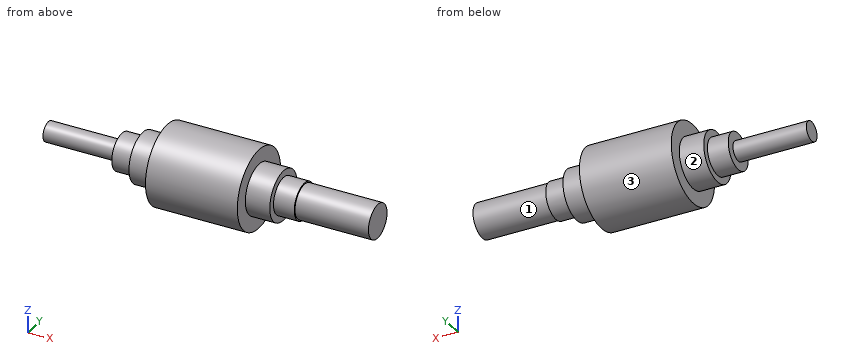
from build123d import *


with BuildPart() as part:
    # Çizim1 → Döndür1 (revolve)
    with BuildSketch(Plane.XY, mode=Mode.PRIVATE) as d_nd_r1_sk:
        Polygon((30, 7.5), (38.5, 7.5), (38.5, 10.25), (48.5, 10.25), (48.5, 16.275), (86, 16.275), (86, 10.25), (96, 10.25), (96, 7.5), (104.5, 7.5), (104.5, 6.975), (134.5, 6.975), (134.5, 0), (0, 0), (0, 4), (30, 4), align=None)
    revolve(d_nd_r1_sk.sketch.rotate(Axis((0, 0, 0), (1, 0, 0)), 90), axis=Axis((0, 0, 0), (1, 0, 0)))


solid = part.part
Work out the finished part from the listing and answer in its coordinate system (mm). Face numbers are marked on the shaded views. A direction names the side the tool comes from. Round coordinates to 2 decimals unless told otherwise and drop trailing zeros. Write each loop counter-clockwise with the first axis right and the second up, starting at its lowest first coordinate (ties: lowest second). Pieces come first, ordered by that corner, then holes. Notation, with made-up numbers: (44.5, 73.25) -> (97.5, 73.25) arc R21 ccw to (97.5, 77.25) -> close; hole circle Ø11 at (3, 75). An arc over 180 degrees is marked (long way). Answer as CSV lines item,"result". Start each with the question number.
(1) The part is cut by section C-C, the plane x = 66. Give the vertices of the cut face in (y, z) (3 decimals).
(2) A tool of negligible diameter and unlimited length cuts with its end or side. For the marked faces 1, 2 and 3, from which of +Z, -Z, +X, -X, +Y, -Y can it reach the whole face along a straight path? Write none if from no direction.
(3) Each of these flat-tipped pins is pushed along its axis until it touches: pin 1 (1.5 mm diameter, centred on y = -10.5, z = 13, fed in from -X); pin 2 (8 mm diameter, centred on x = 51, z = -8, fed in from -Y); pin 3 (2 mm diameter, centred on y = 11.5, z = 2, fed in from +X). Where does it stop, or does it pass through?
(4) The part is cut by section A-A, the plane z = 0. Give the vertices of the cut face in (x, y) (3 decimals).
(5) Find the intervals of material crossed by probe 1 along X at (y, z) = (11, 5.5); probe 2 along X at (y, z) = (-5, -1); probe 3 along Z at (x, y) = (116.5, -0.5), in increasing order.
(6) The part is cut by section D-D, the plane z = 5.5. Give the vertices of the cut face in (x, y), then the cut area to 3 significant figures.
Output values:
1,outline,"circle Ø32.55 at (0, 0)"
2,face 1,"+X"
2,face 2,"-X"
2,face 3,"+X, -X"
3,pin 1,"stops at x = 48.5"
3,pin 2,"stops at y = -15.78"
3,pin 3,"stops at x = 86"
4,outline,"(0, -4) -> (30, -4) -> (30, -7.5) -> (38.5, -7.5) -> (38.5, -10.25) -> (48.5, -10.25) -> (48.5, -16.275) -> (86, -16.275) -> (86, -10.25) -> (96, -10.25) -> (96, -7.5) -> (104.5, -7.5) -> (104.5, -6.975) -> (134.5, -6.975) -> (134.5, 6.975) -> (104.5, 6.975) -> (104.5, 7.5) -> (96, 7.5) -> (96, 10.25) -> (86, 10.25) -> (86, 16.275) -> (48.5, 16.275) -> (48.5, 10.25) -> (38.5, 10.25) -> (38.5, 7.5) -> (30, 7.5) -> (30, 4) -> (0, 4) -> close"
5,probe 1,"x = 48.5 to 86"
5,probe 2,"x = 30 to 134.5"
5,probe 3,"z = -6.96 to 6.96"
6,outline,"(30, -5.1) -> (38.5, -5.1) -> (38.5, -8.65) -> (48.5, -8.65) -> (48.5, -15.32) -> (86, -15.32) -> (86, -8.65) -> (96, -8.65) -> (96, -5.1) -> (104.5, -5.1) -> (104.5, -4.29) -> (134.5, -4.29) -> (134.5, 4.29) -> (104.5, 4.29) -> (104.5, 5.1) -> (96, 5.1) -> (96, 8.65) -> (86, 8.65) -> (86, 15.32) -> (48.5, 15.32) -> (48.5, 8.65) -> (38.5, 8.65) -> (38.5, 5.1) -> (30, 5.1) -> close"
6,area,"1,930 mm²"
